Could you check a few things on this model? Use its own coordinates, in mm. Give positions to 0.01 mm unless a question says otherwise; leave off trailing zeros. Order: outer loops, then holes, each group sorted by start corner. A loop starts at its lowest first (then second) coordinate and runs counter-clockwise, first axis right, second up.
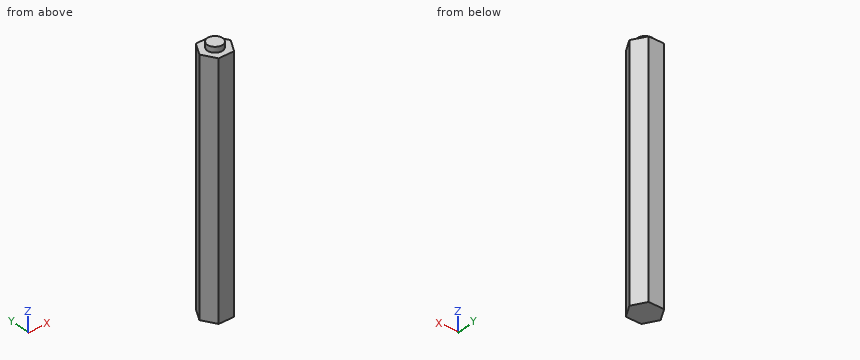
Autodesk Inventor part; units mm, degrees
ref_plane "YZ Plane" through (0, 0, 0) normal (1, 0, 0) x (0, 1, 0)
ref_plane "XZ Plane" through (0, 0, 0) normal (0, 1, 0) x (-1, 0, 0)
ref_plane "XY Plane" through (0, 0, 0) normal (0, 0, 1) x (1, 0, 0)
sketch "Sketch1" plane through (0, 0, 0) normal (0, 0, 1) x (1, 0, 0)
  line L0 (-3.7629, 6.2932) -> (3.5686, 6.4054)
  line L1 (3.5686, 6.4054) -> (7.3315, 0.1122)
  line L2 (7.3315, 0.1122) -> (3.7629, -6.2932)
  line L3 (3.7629, -6.2932) -> (-3.5686, -6.4054)
  line L4 (-3.5686, -6.4054) -> (-7.3315, -0.1122)
  line L5 (-7.3315, -0.1122) -> (-3.7629, 6.2932)
  point P0 (0, 0)
  point P1 (0, 0)
  dimension "d0" = 12.7
extrude "Extrusion1" add sketch "Sketch1" along normal blind 101.6
sketch "Sketch2" plane through (0, 0, 101.6) normal (0, 0, 1) x (1, 0, 0)
  circle A0 centre (0, 0) radius 4.1084
extrude "Extrusion2" add sketch "Sketch2" along normal blind 0.254
sketch "Sketch3" plane through (0, 0, 101.6) normal (0, 0, 1) x (1, 0, 0)
  line L0 (3.5686, 6.4054) -> (-3.7629, 6.2932)
  line L1 (-3.7629, 6.2932) -> (-7.3315, -0.1122)
  line L2 (-7.3315, -0.1122) -> (-3.5686, -6.4054)
  line L3 (-3.5686, -6.4054) -> (3.7629, -6.2932)
  line L4 (3.7629, -6.2932) -> (7.3315, 0.1122)
  line L5 (7.3315, 0.1122) -> (3.5686, 6.4054)
extrude "Extrusion3" add sketch "Sketch3" along normal blind 12.7
sketch "Sketch4" plane through (0, 0, 114.3) normal (0, 0, 1) x (1, 0, 0)
  circle A0 centre (0, 0) radius 3.5518
extrude "Extrusion4" add sketch "Sketch4" along normal blind 2.54
properties part number "4.5 hex shaft" material "Aluminum 6061"
Item 1: Imagine slicing it at C-C on x = 1.5. List the corners of the cut face in (y, z) for me.
Findings:
outline: (-6.33, 0) - (6.37, 0) - (6.37, 114.3) - (3.22, 114.3) - (3.22, 116.84) - (-3.22, 116.84) - (-3.22, 114.3) - (-6.33, 114.3) - close
Item 2: Please list where these lines run through material, in increasing order: line 1 along Y through (x, z) = (-3, 13); line 2 along Z through (x, y) = (-4.75, 2.5); line 3 along Y through (x, z) = (5.5, 15).
Findings:
line 1: y = -6.4 to 6.3
line 2: z = 0 to 114.3
line 3: y = -3.18 to 3.18
Item 3: For pin 1 (6 mm diameter, centred on x = 4, y = -2.5, fed in from -Z); pin 2 (1.5 mm diameter, centred on y = 2.5, z = 95.5, fed in from +X); pin 3 (3 mm diameter, centred on y = 4.5, z = 20, fed in from -X); pin 4 (4 mm diameter, centred on y = 5, z = 85.5, fed in from +X), each with a flat end and sliding along its axis, tell me the tip position at first contact or that it passes through.
Findings:
pin 1: stops at z = 0
pin 2: stops at x = 6.35
pin 3: stops at x = -5.6
pin 4: stops at x = 5.6
Item 4: Imagine slicing it at D-D on x = -5. List the corners of the cut face in (y, z) for me, then the cut area to 3 significant figures.
Findings:
outline: (-4.01, 0) - (4.07, 0) - (4.07, 114.3) - (-4.01, 114.3) - close
area: 924 mm2
Item 5: Imagine slicing it at A-A on z = 86. List the corners of the cut face in (x, y) for me.
Findings:
outline: (-7.33, -0.11) - (-3.57, -6.41) - (3.76, -6.29) - (7.33, 0.11) - (3.57, 6.41) - (-3.76, 6.29) - close
Item 6: Imagine slicing it at B-B on y = 1.5. List the corners of the cut face in (x, z) for me.
Findings:
outline: (-6.43, 0) - (6.5, 0) - (6.5, 114.3) - (3.22, 114.3) - (3.22, 116.84) - (-3.22, 116.84) - (-3.22, 114.3) - (-6.43, 114.3) - close
